Read the model definition and answer for the solid it produces. Units are mm, in the model's axes. Face numbers are marked on the shaded views. A direction names the side the tool comes from. Round coordinates to 2 decimals unless told otherwise and drop trailing zeros. Order: outer loops, then holes, each group sorted by start corner. A loop starts at its lowest first (then second) coordinate and runs counter-clockwise, first axis right, second up.
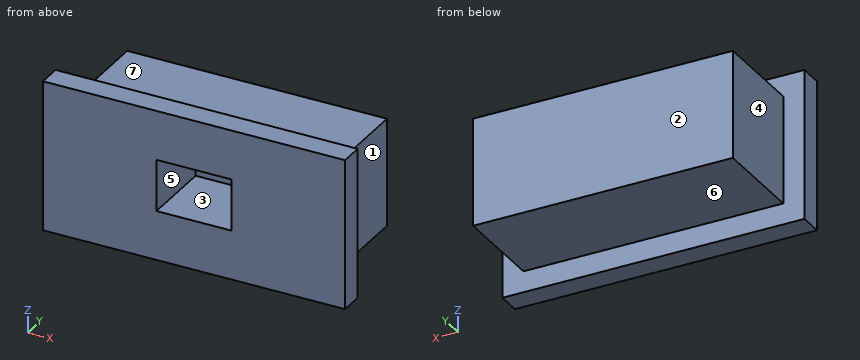
from build123d import *

# Parameters (mm, degrees)
SKETCH1_W           = 12.88
SKETCH1_H           = 6.4
BOSS_EXTRUDE1_DEPTH = 1
SKETCH3_W           = 11.08
SKETCH3_H           = 4.6
BOSS_EXTRUDE2_DEPTH = 4
SKETCH4_W           = 3.2
SKETCH4_H           = 2.2
CUT_EXTRUDE1_DEPTH  = 3.1


with BuildPart() as part:
    # Sketch1 → Boss-Extrude1 (new body)
    with BuildSketch(Plane(origin=(0, 0, 0), x_dir=(1, 0, 0), z_dir=(0, 1, 0))):
        with Locations((6.44, 3.2)):
            Rectangle(SKETCH1_W, SKETCH1_H)
    extrude(amount=BOSS_EXTRUDE1_DEPTH)

    # Sketch3 → Boss-Extrude2 (add)
    with BuildSketch(Plane(origin=(0, 1, 0), x_dir=(1, 0, 0), z_dir=(0, 1, 0))):
        with Locations((6.44, 3.2)):
            Rectangle(SKETCH3_W, SKETCH3_H)
    extrude(amount=BOSS_EXTRUDE2_DEPTH)

    # Sketch4 → Cut-Extrude1 (cut)
    with BuildSketch(Plane.XZ):
        with Locations((6.44, -3.2)):
            Rectangle(SKETCH4_W, SKETCH4_H)
    extrude(amount=-CUT_EXTRUDE1_DEPTH, mode=Mode.SUBTRACT)


solid = part.part
Q1. For the marked faces 4, 5, 6 and 7, determine the directions among +Z, -Z, +X, -X, +Y, -Y from which every point of the face is accessible in a straight line to the end or side of a thin tool.
Outcome:
face 4: +Z, -Z, -X, +Y
face 5: -Y
face 6: -Z, +X, -X, +Y
face 7: +Z, +X, -X, +Y
Q2. A cutting plane is placed at D-D, the plane z = -5. Give the vertices of the cut face in (x, y), plus the area to 3 significant figures.
Outcome:
outline: (0, 0) - (12.88, 0) - (12.88, 1) - (11.98, 1) - (11.98, 5) - (0.9, 5) - (0.9, 1) - (0, 1) - close
area: 57.2 mm2
Q3. Flat-ended cylindrical pins translate along their axes: pin 1 (2 mm diameter, centred on y = 3, z = -3.5, fed in from +X); pin 2 (1.2 mm diameter, centred on x = 5, y = 4, fed in from -Z); pin 3 (1.2 mm diameter, centred on y = 3, z = -3.5, fed in from -X). Find the tip coordinate at first contact, or state that the pin passes through.
Outcome:
pin 1: stops at x = 11.98
pin 2: stops at z = -5.5
pin 3: stops at x = 0.9
Q4. A cutting plane is placed at A-A, the plane y = 0.8. Give the vertices of the cut face in (x, z), plus the area to 3 significant figures.
Outcome:
outline: (0, -6.4) - (12.88, -6.4) - (12.88, 0) - (0, 0) - close; hole (4.84, -4.3) - (8.04, -4.3) - (8.04, -2.1) - (4.84, -2.1) - close
area: 75.4 mm2
Q5. A cutting plane is placed at B-B, the plane z = -2.75. Give the vertices of the cut face in (x, y).
Outcome:
outline: (0, 0) - (4.84, 0) - (4.84, 3.1) - (8.04, 3.1) - (8.04, 0) - (12.88, 0) - (12.88, 1) - (11.98, 1) - (11.98, 5) - (0.9, 5) - (0.9, 1) - (0, 1) - close
Q6. A cutting plane is placed at C-C, the plane x = 5.25. Give the vertices of the cut face in (y, z), plus the area to 3 significant figures.
Outcome:
outline: (0, -6.4) - (1, -6.4) - (1, -5.5) - (5, -5.5) - (5, -0.9) - (1, -0.9) - (1, 0) - (0, 0) - (0, -2.1) - (3.1, -2.1) - (3.1, -4.3) - (0, -4.3) - close
area: 18.0 mm2
Q7. For a pull along X with two mould halves and no side action, classify the marked faces 1, 2 and 3 as released by +X, released by -X, zero draft, split by the parting line, or undercut.
Outcome:
face 1: released by +X
face 2: zero draft
face 3: undercut
Q8. Straight lines are drawn through the part: probe 1 along X at (y, z) = (1.55, -3.5); probe 2 along X at (y, z) = (1.8, -1.5); probe 3 along Z at (x, y) = (2, 3.55). For each, find the intervals that lie inside material, in ascending order.
Outcome:
probe 1: x = 0.9 to 4.84, 8.04 to 11.98
probe 2: x = 0.9 to 11.98
probe 3: z = -5.5 to -0.9
